Geometry check sheet. Reference: the model listing, model coordinates, mm. Round coordinates to 2 decimals unless told otherwise and drop trailing zeros. Write each loop counter-clockwise with the first axis right and the second up, starting at its lowest first coordinate (ties: lowest second). Pieces come first, ordered by that corner, then holes. Notation, with made-up numbers: (-24, 57) -> (2, 57) arc R27 cw to (2, 73) -> close; hole circle Ø9 at (59.25, 88.25). An arc over 180 degrees is marked (long way). One line per question, with ' | ' between items.
```python
from build123d import *

# Parameters (mm, degrees)
SKETCH2_R           = 11.1125
SKETCH2_R_2         = 2.4892
SKETCH2_R_3         = 22.225
BOSS_EXTRUDE1_DEPTH = 3.175


with BuildPart() as part:
    # Sketch2 → Boss-Extrude1 (new body)
    with BuildSketch(Plane.XY):
        with BuildLine():
            Line((-142.632381685, -29.937060043), (-142.632381685, -64.77))
            ThreePointArc((-142.632381685, -64.77), (-141.144484133, -68.362102448), (-137.552381685, -69.85))
            Line((-137.552381685, -69.85), (137.552381685, -69.85))
            ThreePointArc((137.552381685, -69.85), (141.144484133, -68.362102448), (142.632381685, -64.77))
            Line((142.632381685, -64.77), (142.632381685, -29.937060043))
            Line((142.632381685, -29.937060043), (142.632381685, 122.462939957))
            ThreePointArc((142.632381685, 122.462939957), (134.600001748, 148.101160684), (108.918256203, 140.209048469))
            Line((108.918256203, 140.209048469), (31.75, 0))
            ThreePointArc((31.75, 0), (0, -31.75), (-31.75, 0))
            Line((-31.75, 0), (-108.918256203, 140.209048469))
            ThreePointArc((-108.918256203, 140.209048469), (-134.600001748, 148.101160684), (-142.632381685, 122.462939957))
            Line((-142.632381685, 122.462939957), (-142.632381685, -29.937060043))
        make_face()
        with Locations((-60.484532313, 12.7)):
            Circle(SKETCH2_R, mode=Mode.SUBTRACT)
        with Locations((-125.726814921, 131.243846084)):
            Circle(SKETCH2_R, mode=Mode.SUBTRACT)
        with Locations((125.726814921, 131.243846084)):
            Circle(SKETCH2_R, mode=Mode.SUBTRACT)
        with Locations((-101.9175, -57.15)):
            Circle(SKETCH2_R_2, mode=Mode.SUBTRACT)
        with Locations((60.484532313, 12.7)):
            Circle(SKETCH2_R, mode=Mode.SUBTRACT)
        with Locations((-89.2175, -57.15)):
            Circle(SKETCH2_R_2, mode=Mode.SUBTRACT)
        with Locations((-76.5175, -57.15)):
            Circle(SKETCH2_R_2, mode=Mode.SUBTRACT)
        with Locations((-63.8175, -57.15)):
            Circle(SKETCH2_R_2, mode=Mode.SUBTRACT)
        with Locations((-51.1175, -57.15)):
            Circle(SKETCH2_R_2, mode=Mode.SUBTRACT)
        with Locations((-38.4175, -57.15)):
            Circle(SKETCH2_R_2, mode=Mode.SUBTRACT)
        with Locations((-25.7175, -57.15)):
            Circle(SKETCH2_R_2, mode=Mode.SUBTRACT)
        with Locations((-13.0175, -57.15)):
            Circle(SKETCH2_R_2, mode=Mode.SUBTRACT)
        with Locations((-0.3175, -57.15)):
            Circle(SKETCH2_R_2, mode=Mode.SUBTRACT)
        with Locations((12.3825, -57.15)):
            Circle(SKETCH2_R_2, mode=Mode.SUBTRACT)
        with Locations((25.0825, -57.15)):
            Circle(SKETCH2_R_2, mode=Mode.SUBTRACT)
        with Locations((37.7825, -57.15)):
            Circle(SKETCH2_R_2, mode=Mode.SUBTRACT)
        with Locations((50.4825, -57.15)):
            Circle(SKETCH2_R_2, mode=Mode.SUBTRACT)
        with Locations((63.1825, -57.15)):
            Circle(SKETCH2_R_2, mode=Mode.SUBTRACT)
        with Locations((75.8825, -57.15)):
            Circle(SKETCH2_R_2, mode=Mode.SUBTRACT)
        with Locations((88.5825, -57.15)):
            Circle(SKETCH2_R_2, mode=Mode.SUBTRACT)
        with Locations((101.2825, -57.15)):
            Circle(SKETCH2_R_2, mode=Mode.SUBTRACT)
        with Locations((-106.68, -9.525)):
            Circle(SKETCH2_R_3, mode=Mode.SUBTRACT)
        with Locations((106.68, -9.525)):
            Circle(SKETCH2_R_3, mode=Mode.SUBTRACT)
    extrude(amount=BOSS_EXTRUDE1_DEPTH)


solid = part.part
```
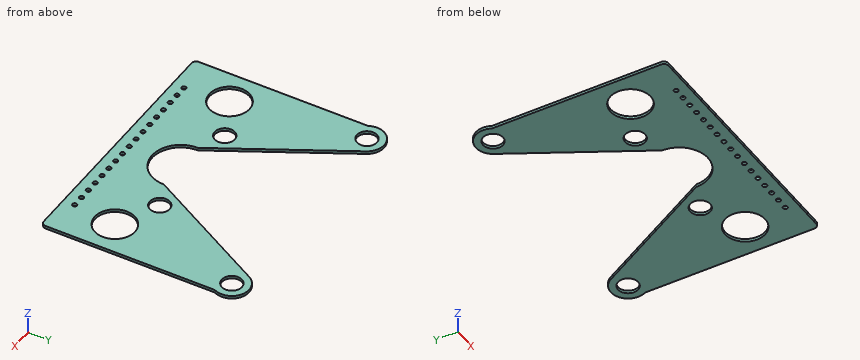
(1) Sectioned sample at B-B on y = 128. Record the cut outline in (x, z) (3 decimals), then the cut area to 3 significant figures.
Resolved:
outline: (-144.499, 0) -> (-136.355, 0) -> (-136.355, 3.175) -> (-144.499, 3.175) -> close; (-115.098, 0) -> (-102.199, 0) -> (-102.199, 3.175) -> (-115.098, 3.175) -> close; (102.199, 0) -> (115.098, 0) -> (115.098, 3.175) -> (102.199, 3.175) -> close; (136.355, 0) -> (144.499, 0) -> (144.499, 3.175) -> (136.355, 3.175) -> close | area: 134 mm2
(2) Sectioned sample at A-A on y = 76. Record the cut outline in (x, z) (3 decimals).
Resolved:
outline: (-142.632, 0) -> (-73.579, 0) -> (-73.579, 3.175) -> (-142.632, 3.175) -> close; (73.579, 0) -> (142.632, 0) -> (142.632, 3.175) -> (73.579, 3.175) -> close
(3) Sectioned sample at C-C on z = 1.85. Count the separate pieces of the cut face and the enclosed holes in it, then the cut area to 3 significant figures.
Resolved:
separate pieces: 1 | enclosed holes: 23 | area: 34,200 mm2
(4) Material ranges on line 1 (Y direction, x = -62, z = 2.75); line 2 (Y direction, x = 120.5, z = 2.4); line 3 (X direction, y = -50, z = 1.95), recorded low to high.
Resolved:
line 1: y = -69.85 to -58.85, -55.45 to 1.69, 23.71 to 54.96 | line 2: y = -69.85 to -26.93, 7.88 to 121.44, 141.05 to 149.56 | line 3: x = -142.63 to 142.63
(5) Go/stop test with flat-tipped pins: pin 1 (3 mm diameter, centred on x = 25.08, y = -57.15, fed in from -Z); pin 2 (1 mm diameter, centred on y = 116.5, z = 1, fed in from -X). Record where each tip stops, or that it passes through.
Resolved:
pin 1: passes through | pin 2: stops at x = -142.63
